Here's how the part is built. I have some questions about the finished solid (model axes, mm). Face numbers are marked on the shaded views. A direction names the side the tool comes from. Round coordinates to 2 decimals unless told otherwise and drop trailing zeros. Write each loop counter-clockwise with the first axis right and the second up, starting at its lowest first coordinate (ties: lowest second). Pieces come first, ordered by that corner, then holes. Notation, with made-up numbers: M -39,10 L 4,10 A28 ccw 4,30 Z; hole C -38,52 d11. An arc over 180 degrees is marked long. Use one line per item in the form item = value. Start each with the question number.
Q1. I need wall thicknesses on line 1 along Y through (x, z) = (-5.5, 18); line 2 along Y through (x, z) = (3.5, 32.5); line 3 along X through (y, z) = (-7.5, 33.5). Which ranges of each line are inside material? Lowest first, please. Write a range as from..to.
Q2. I'm going to push a flat-ended pin straight in: pin 1 Ø8 at (x, y) = (1, 9.5) entering from -Z. Where does the tip first touch, or does it pass through?
Q3. I want a section at A-A on x = 2. List the corners of the cut face in (y, z) for me, and give its area (3 significant figures).
Q4. I want a section at B-B on y = -3. List the corners of the cut face in (x, z) for me (3 decimals), and give its area (3 significant figures).
Q5. We'd pull the mould along Y, two halves only. Please class the marked faces 3, 4 and 5: +Y half, -Y half, draft (parallel to the pull), parting line (faces both ways), or undercut.
Q6. For the marked faces 1 and 2, which set-ups out of +Z, -Z, +X, -X, +Y, -Y let a thin tool reach every point of the face, with its end or its side?
```python
from build123d import *

# Parameters (mm, degrees)
SKETCH_R             = 10.15
PAD_DEPTH            = 35.4
SKETCH001_W          = 1.455354
SKETCH001_H          = 0.628309
POCKET_DEPTH         = 148.624187
POLARPATTERN_COUNT   = 8
FILLET_R             = 2
SKETCH002_R          = 7
POCKET001_DEPTH      = 21.426335
POCKET001_DEPTH_BACK = 22.734483
FILLET001_R          = 1


with BuildPart() as part:
    # Sketch → Pad (new body)
    with BuildSketch(Plane.XY):
        with BuildLine():
            Line((-16.075, 12.15), (-16.075, -12.15))
            ThreePointArc((-16.075, -12.15), (-15.19632, -14.27132), (-13.075, -15.15))
            Line((-13.075, -15.15), (13.075, -15.15))
            ThreePointArc((13.075, -15.15), (15.19632, -14.27132), (16.075, -12.15))
            Line((16.075, -12.15), (16.075, 12.15))
            ThreePointArc((16.075, 12.15), (15.19632, 14.27132), (13.075, 15.15))
            Line((13.075, 15.15), (-13.075, 15.15))
            ThreePointArc((-13.075, 15.15), (-15.19632, 14.27132), (-16.075, 12.15))
        make_face()
        Circle(SKETCH_R, mode=Mode.SUBTRACT)
    extrude(amount=PAD_DEPTH)

    # Sketch001 (on Face11 of Pad) → Pocket (cut, through all)
    with BuildSketch(Plane.XY.offset(35.4)):
        with Locations((0, 10.060702)):
            Rectangle(SKETCH001_W, SKETCH001_H)
    pocket = extrude(amount=-POCKET_DEPTH, mode=Mode.SUBTRACT)

    # PolarPattern: Pocket ×8 about axis
    polarpattern_axis = Axis((0, 0, 35.4), (0, 0, 1))
    for i in range(1, POLARPATTERN_COUNT):
        add(pocket.rotate(polarpattern_axis, i * 360 / POLARPATTERN_COUNT), mode=Mode.SUBTRACT)

    # Fillet
    fillet_edges = [part.edges().sort_by_distance(p)[0] for p in [
        (-16.075, 0, 35.4),
    ]]
    fillet(fillet_edges, radius=FILLET_R)

    # Sketch002 (on DatumPlane) → Pocket001 (cut, two sides)
    with BuildSketch(Plane(origin=(-14.984859, 14.059859, 16.7), x_dir=(-0.707107, 0.707107, 0), z_dir=(0.707107, 0.707107, 0))) as pocket001_sk:
        with Locations((2.048201, 0)):
            Circle(SKETCH002_R)
    extrude(amount=-POCKET001_DEPTH, mode=Mode.SUBTRACT)
    extrude(pocket001_sk.sketch, amount=POCKET001_DEPTH_BACK, mode=Mode.SUBTRACT)

    # Fillet001
    fillet001_edges = [part.edges().sort_by_distance(p)[0] for p in [
        (-6.891817, 15.15, 16.7),
    ]]
    fillet(fillet001_edges, radius=FILLET001_R)


solid = part.part
```
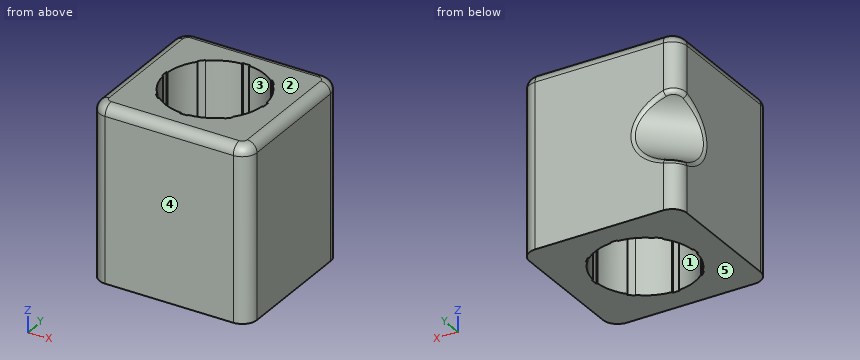
Reported:
q1.line_1 = -15.15..-8.53, 8.53..15.15
q1.line_2 = -15.15..-9.53, 9.53..15.15
q1.line_3 = -16.07..-7.17, 7.17..16.07
q2.pin_1 = 0
q3.outline = M -15.15,0 L -9.95,0 L -9.95,35.4 L -13.15,35.4 A2 ccw -15.15,33.4 Z; M 9.95,0 L 15.15,0 L 15.15,33.4 A2 ccw 13.15,35.4 L 9.95,35.4 Z
q3.area = 366 mm^2
q4.outline = M -16.075,0 L -9.697,0 L -9.697,35.4 L -14.075,35.4 A2 ccw -16.075,33.4 Z; M 9.697,0 L 16.075,0 L 16.075,33.4 A2 ccw 14.075,35.4 L 9.697,35.4 Z
q4.area = 450 mm^2
q5.face_3 = undercut
q5.face_4 = -Y half
q5.face_5 = draft
q6.face_1 = +Z, -Z
q6.face_2 = +Z, +X, -X, +Y, -Y
